Can you work these out from the model? Positions are in its coordinate system, mm. A direction names the side the tool comes from. Round coordinates to 2 decimals unless told otherwise and drop trailing zeros. Loops run counter-clockwise (first coordinate to the right, second up) from the corner with the lowest first, then second, coordinate; pieces in that order, holes last. Notation, with made-up numbers: (77.5, 16.5) - (102.5, 16.5) arc R18 cw to (102.5, 27.5) - close; hole circle Ø7 at (37.25, 2.25). An arc over 180 degrees is marked (long way). Answer as CSV lines item,"result".
```python
from build123d import *

# Parameters (mm, degrees)
F1_DEPTH = 120
F3_DEPTH = 117
F5_DEPTH = 118.5
F8_R     = 2.5
F9_DEPTH = 25


with BuildPart() as f1:
    # F0 (on Front) → F1 (new body)
    with BuildSketch(Plane.XZ):
        with BuildLine():
            ThreePointArc((0, -35), (35, 0), (0, 35))
            Line((0, 35), (0, -35))
        make_face()
    extrude(amount=F1_DEPTH)

    # F2 (on face) → F3 (cut)
    with BuildSketch(Plane.XZ.offset(120)):
        with BuildLine():
            ThreePointArc((0, -32), (32, 0), (0, 32))
            Line((0, 32), (0, -32))
        make_face()
    extrude(amount=-F3_DEPTH, mode=Mode.SUBTRACT)

    # F4 (on face) → F5 (cut)
    with BuildSketch(Plane.XZ.offset(120)):
        with BuildLine():
            ThreePointArc((3, 31.8590646441), (2.0009811174, 31.9373773903), (1, 31.9843711834))
            Line((1, 31.9843711834), (1, -31.9843711834))
            ThreePointArc((1, -31.9843711834), (2.0009811174, -31.9373773903), (3, -31.8590646441))
            Line((3, -31.8590646441), (3, 31.8590646441))
        make_face()
        with BuildLine():
            Line((3, 33.5), (1, 33.5))
            Line((1, 33.5), (1, 31.9843711834))
            ThreePointArc((1, 31.9843711834), (2.0009811174, 31.9373773903), (3, 31.8590646441))
            Line((3, 31.8590646441), (3, 33.5))
        make_face()
        with BuildLine():
            ThreePointArc((3, -31.8590646441), (2.0009811174, -31.9373773903), (1, -31.9843711834))
            Line((1, -31.9843711834), (1, -33.5))
            Line((1, -33.5), (3, -33.5))
            Line((3, -33.5), (3, -31.8590646441))
        make_face()
    extrude(amount=-F5_DEPTH, mode=Mode.SUBTRACT)

    # F8 (on line) → F9 (cut)
    with BuildSketch(Plane.YZ.offset(35)):
        with Locations((-100, 0)):
            Circle(F8_R)
    extrude(amount=-F9_DEPTH, mode=Mode.SUBTRACT)


solid = f1.part
```
Q1. If I drill on line 1 along Y through (x, z) = (34, 0); line 2 along Y through (x, z) = (5, 6); line 3 along Z through (x, y) = (32, -100), over which ranges is the centre line in solid material (lowest first)? Write a range as [from, to].
Checks:
line 1,"[-120, -102.5], [-97.5, 0]"
line 2,"[-3, 0]"
line 3,"[-14.18, -2.5], [2.5, 14.18]"
Q2. Imagine slicing it at C-C (y = -100). Write out the boundary of the cut face in (x, z), then the cut area to 3 significant figures.
Checks:
outline,"(0, -35) arc R35 ccw to (34.91, -2.5) - (31.9, -2.5) arc R32 cw to (3, -31.86) - (3, -33.5) - (1, -33.5) - (1, -31.98) arc R32 cw to (0, -32) - close; (0, 32) arc R32 cw to (1, 31.98) - (1, 33.5) - (3, 33.5) - (3, 31.86) arc R32 cw to (31.9, 2.5) - (34.91, 2.5) arc R35 ccw to (0, 35) - close"
area,"294 mm²"
Q3. I'm going to push flat-ended pins straight in: pin 1 Ø1 at (x, y) = (21.5, -76.5) entering from -Z; pin 2 Ø6 at (y, z) = (-37, -8) entering from -X; pin 3 Ø1 at (x, y) = (2, -62) entering from +Z; pin 4 Ø1.5 at (x, z) = (24, -20) entering from +Y. Where does each tip first touch, or does it pass through?
Checks:
pin 1,"z = -28"
pin 2,"x = 30.05"
pin 3,"z = 34.97"
pin 4,"y = 0"
Q4. Imagine slicing it at D-D (x = 17). Write out the boundary of the cut face in (y, z).
Checks:
outline,"(-120, -30.59) - (0, -30.59) - (0, 30.59) - (-120, 30.59) - (-120, 27.11) - (-3, 27.11) - (-3, -27.11) - (-120, -27.11) - close"
Q5. Imagine slicing it at B-B (y = -28). Write out the boundary of the cut face in (x, z), then the cut area to 3 significant figures.
Checks:
outline,"(0, -35) arc R35 ccw to (0, 35) - (0, 32) arc R32 cw to (1, 31.98) - (1, 33.5) - (3, 33.5) - (3, 31.86) arc R32 cw to (3, -31.86) - (3, -33.5) - (1, -33.5) - (1, -31.98) arc R32 cw to (0, -32) - close"
area,"309 mm²"
Q6. We'd pull the mould along Z, two halves only. Please class faces 4 (the cylindrical face through (34.99, -59.16, -0.77)), 5 (the cylindrical face through (33.473, -97.615, 0.751)), 6 (the flat face through (13, 0, 0)): pulls with the +Z half, pulls with the -Z half, needs draft (parallel to the pull), parting line crosses it, or undercut.
Checks:
face 4,"parting line crosses it"
face 5,"undercut"
face 6,"needs draft"
Q7. On a 3-axis mill with a long thin cutter (end or side, diameter ignored), from which of +Z, -Z, +X, -X, +Y, -Y can I reach the whole of each face in a straight line? I mean faces 1 (the flat face through (1, -61, 32.4)), 2 (the flat face through (0, -42, -34)), 3 (the cylindrical face through (31.993, -62.319, -0.662)). Say none if no direction works.
Checks:
face 1,"-Y"
face 2,"+Z, -Z, -X, +Y, -Y"
face 3,"-X, -Y"
Q8. Imagine slicing it at A-A (z = 0). Write out the boundary of the cut face in (x, y).
Checks:
outline,"(0, -3) - (1, -3) - (1, -1.5) - (3, -1.5) - (3, -3) - (32, -3) - (32, -97.5) - (35, -97.5) - (35, 0) - (0, 0) - close; (32, -120) - (35, -120) - (35, -102.5) - (32, -102.5) - close"
